Geometry check sheet. Reference: the model listing, model coordinates, mm. A direction names the side the tool comes from. Give positions to 0.01 mm unless a question says otherwise; leave off trailing zeros. One line per question, with ' | ' between items. Start each with the question number.
Q1. Gauge pin test, flat ends, axial feed: P1, Ø12, axis at y = 2, z = 21.5, coming from the +X side; P2, Ø23, axis at x = -5.5, z = 6, coming from the +Y side; P3, Ø13, axis at x = -22.5, y = 20.5, coming from the +Z side; P4, Ø1, axis at x = 16, z = 24, coming from the +Y side. Record the tip position at first contact, or that the pin passes through.
Q2. Release check for a two-part mould opening along X. For faces 1 (the face through (-35.735, 8.761, -2.956)), 2 (the face through (-22.839, 22.415, -0.199)), 3 (the face through (-22.2, 22.3, 15.2)) record: +X half, -X half, draft (parallel to the pull), parting line (faces both ways), or undercut.
Q3. Thickness scan on L1, parallel to Z at x = 14, y = 6.5; L2, parallel to Y at x = -35, z = -12.5; L3, parallel to Z at x = 4.5, y = 22.5. Record the ranges inside material, lowest first. Write a range as [from, to].
Q4. Set-up check for faces 4 (the face through (36.57, -11.24, -4.8)), 5 (the face through (-1, -20, 0)), 6 (the face through (-22.4, 22.1, -14.2)): record each of +Z, -Z, +X, -X, +Y, -Y from which the full face is reachable in a straight line by a thin tool's end or side.
```python
from build123d import *

# Parameters (mm, degrees)
CUT_EXTRUDE1_DEPTH      = 70.282032303
CUT_EXTRUDE1_DEPTH_BACK = 70.282032303
SKETCH3_W               = 80
SKETCH3_H               = 50
CUT_EXTRUDE2_DEPTH      = 70.282032303
CUT_EXTRUDE2_DEPTH_BACK = 70.282032303
CUT_EXTRUDE3_DEPTH      = 1
SKETCH6_R               = 1
CUT_EXTRUDE4_DEPTH      = 1
FILLET1_R               = 2
SKETCH7_W               = 3
SKETCH7_H               = 1.5
FILLET2_R               = 2


with BuildPart() as part:
    # Sketch2 → Revolve4 (revolve)
    with BuildSketch(Plane(origin=(0, 0, 0), x_dir=(0, 0, -1), z_dir=(1, 0, 0))):
        with BuildLine():
            Line((0, 40), (0, -40))
            ThreePointArc((0, -40), (-40, 0), (0, 40))
        make_face()
    revolve(axis=Axis((0, 0, 0), (0, 1, 0)))

    # Sketch3 → Cut-Extrude1 (cut, two sides: drawn at the far end of the back side and taken through both)
    with BuildSketch(Plane.XY.offset(-CUT_EXTRUDE1_DEPTH_BACK)):
        with Locations((0, -45)):
            Rectangle(SKETCH3_W, SKETCH3_H)
    extrude(amount=CUT_EXTRUDE1_DEPTH + CUT_EXTRUDE1_DEPTH_BACK, mode=Mode.SUBTRACT)

    # Sketch4 → Cut-Extrude2 (cut, two sides: drawn at the far end of the back side and taken through both)
    with BuildSketch(Plane.XY.offset(-CUT_EXTRUDE2_DEPTH_BACK)):
        Polygon((-40.264401604, 4.909155965), (-4.990432392, 40.34567803), (-21.331481222, 54.070064096), (-80.21701071, 4.909155965), align=None)
    extrude(amount=CUT_EXTRUDE2_DEPTH + CUT_EXTRUDE2_DEPTH_BACK, mode=Mode.SUBTRACT)

    # Sketch5 → Cut-Extrude3 (cut)
    with BuildSketch(Plane(origin=(-22.679314195, 22.575280643, 0), x_dir=(0, 0, 1), z_dir=(-0.708730441300506, 0.705479384230319, 0))):
        with BuildLine():
            Line((15.2, 11.2), (15.2, -11.2))
            ThreePointArc((15.2, -11.2), (13.442640687, -15.442640687), (9.2, -17.2))
            Line((9.2, -17.2), (-9.2, -17.2))
            ThreePointArc((-9.2, -17.2), (-13.442640687, -15.442640687), (-15.2, -11.2))
            Line((-15.2, -11.2), (-15.2, 11.2))
            ThreePointArc((-15.2, 11.2), (-13.442640687, 15.442640687), (-9.2, 17.2))
            Line((-9.2, 17.2), (9.2, 17.2))
            ThreePointArc((9.2, 17.2), (13.442640687, 15.442640687), (15.2, 11.2))
        make_face()
        with BuildLine():
            Line((-9.2, 16.2), (9.2, 16.2))
            ThreePointArc((9.2, 16.2), (12.735533906, 14.735533906), (14.2, 11.2))
            Line((14.2, 11.2), (14.2, -11.2))
            ThreePointArc((14.2, -11.2), (12.735533906, -14.735533906), (9.2, -16.2))
            Line((9.2, -16.2), (-9.2, -16.2))
            ThreePointArc((-9.2, -16.2), (-12.735533906, -14.735533906), (-14.2, -11.2))
            Line((-14.2, -11.2), (-14.2, 11.2))
            ThreePointArc((-14.2, 11.2), (-12.735533906, 14.735533906), (-9.2, 16.2))
        make_face(mode=Mode.SUBTRACT)
    extrude(amount=-CUT_EXTRUDE3_DEPTH, mode=Mode.SUBTRACT)

    # Sketch6 → Cut-Extrude4 (cut)
    with BuildSketch(Plane(origin=(-22.679314195, 22.575280643, 0), x_dir=(0, 0, 1), z_dir=(-0.708730441300506, 0.705479384230319, 0))):
        with Locations(Location((0, -20, 0), (0, 0, 270))):
            Circle(SKETCH6_R)
        with Locations(Location((3, -20, 0), (0, 0, 270))):
            Circle(SKETCH6_R)
        with Locations(Location((6, -20, 0), (0, 0, 270))):
            Circle(SKETCH6_R)
        with Locations(Location((-3, -20, 0), (0, 0, 270))):
            Circle(SKETCH6_R)
        with Locations(Location((-6, -20, 0), (0, 0, 270))):
            Circle(SKETCH6_R)
    extrude(amount=-CUT_EXTRUDE4_DEPTH, mode=Mode.SUBTRACT)

    # Fillet1
    fillet1_edges = [part.edges().sort_by_distance(p)[0] for p in [
        (-5.747729438, 39.584891137, 0),
    ]]
    fillet(fillet1_edges, radius=FILLET1_R)

    # Sketch7 → Cut-Revolve1 (revolve, cut)
    with BuildSketch(Plane(origin=(0, 0, 0), x_dir=(0, 0, -1), z_dir=(1, 0, 0))):
        with Locations((-38.385381332, -11.25)):
            Rectangle(SKETCH7_W, SKETCH7_H)
    revolve(axis=Axis((0, 0, 0), (0, 1, 0)), mode=Mode.SUBTRACT)

    # Fillet2
    fillet2_edges = [part.edges().sort_by_distance(p)[0] for p in [
        (0, -20, -34.641016151),
    ]]
    fillet(fillet2_edges, radius=FILLET2_R)


solid = part.part
```
Working result:
1) P1: stops at x = 36.84 | P2: stops at y = 40 | P3: stops at z = 32.05 | P4: stops at y = 28.22
2) face 1: undercut | face 2: -X half | face 3: draft
3) L1: z = [-36.9, 36.9] | L2: y = [-14.79, -12], [-10.5, 10.2] | L3: z = [-32.76, 32.76]
4) face 4: none | face 5: +Z, -Z, +X, -X, -Y | face 6: -X, +Y
